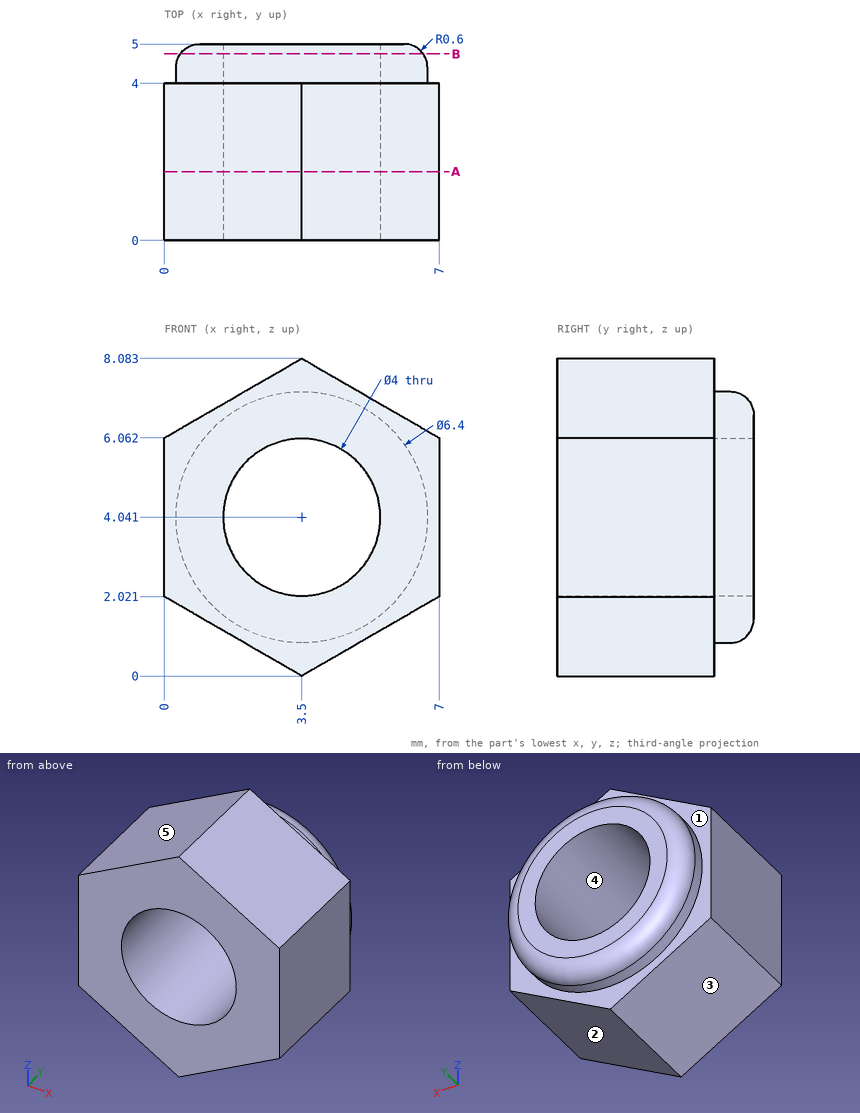
For this review, use the dimensioned drawing (mm, ordinates from the lowest corner) and the shaded views. A direction names the side the tool comes from. Give positions to 0.01 mm unless a question says otherwise; leave off trailing zeros. Loops run counter-clockwise (first coordinate to the right, second up) from the corner with the lowest first, then second, coordinate; pieces in that order, holes last. Notation, with made-up numbers: (-18, 33.5) -> (20, 33.5) arc R12 ccw to (20, 37.5) -> close; hole circle Ø11 at (-37.5, 0). An arc over 180 degrees is marked (long way). One line per question, with ' | ' between items. Start each with the question number.
(1) We need section A-A (y = 1.75). State the section outline as (x, z) points.
(2) For line 1 (Z direction, x = 6, y = 3.1) (1 decimal); line 2 (Y direction, x = 1.5, z = 1.5); line 3 (Z direction, x = 5.25, y = 0.7) (1 decimal), list the stretches that pass through material, from the lowest coordinate up.
(3) We need section B-B (y = 4.75). State the section outline as (x, z) points (1 decimal).
(4) Draft analysis for pull direction Z (two halves, no side actions). For the marked faces 3, 4 and 5, state which applies: +Z half, -Z half, draft (parallel to the pull), parting line (faces both ways), or undercut.
(5) For the marked faces 1 and 2, list the 3-axis set-ups (+Z, -Z, +X, -X, +Y, -Y) from which the entire face can be reached by the end or side of a thin tool; tool diameter is ignored.
(6) Insertion check: P1, Ø1, axis at x = 1.5, y = 1, coming from the -Z side (1 decimal); P2, Ø3, axis at x = 3.5, y = 1.5, coming from the +Z side. Each pin has a flat end and moves straight along its axis. Give the tip position at first contact, or say it passes through.
The answers:
1) outline: (0, 2.02) -> (3.5, 0) -> (7, 2.02) -> (7, 6.06) -> (3.5, 8.08) -> (0, 6.06) -> close; hole circle Ø4 at (3.5, 4.04)
2) line 1: z = 1.4 to 6.6 | line 2: y = 0 to 4 | line 3: z = 1 to 3.1, 5 to 7.1
3) outline: circle Ø6.2 at (3.5, 4); hole circle Ø4 at (3.5, 4)
4) face 3: -Z half | face 4: undercut | face 5: +Z half
5) face 1: +Y | face 2: -Z, +X, +Y, -Y
6) P1: stops at z = 0.9 | P2: stops at z = 8.08
